Model file for the job. Use its own axes, mm. Give positions to 0.01 mm unless a question says otherwise; leave off trailing zeros. Order: outer loops, then holes, each group sorted by start corner. A loop starts at its lowest first (then second) coordinate and runs counter-clockwise, first axis right, second up. Notation, with made-up numbers: (77.5, 5.25) - (126.5, 5.25) arc R18 ccw to (126.5, 20.25) - close; hole circle Ø11 at (-19, -19). An arc over 180 degrees is marked (long way). Use CSV: the item, a comma, the result in double quotes. Start each with the question number.
(1) Band-saw the part on A-A, the plane x = 0. Give the cut face in (y, z), then the cut area to 3 significant figures.
(2) Band-saw the part on B-B, the plane y = -280. Give the cut face in (x, z).
(3) Probe L1, parallel to Y at x = 0, z = 12.5; L2, parallel to X at y = 269.5, z = 15.5; L3, parallel to Y at x = -280, z = 14.75. List the from-to ranges inside material, lowest first.
(4) Drop flat-ended pins along their axis: pin 1 Ø6 at (y, z) = (71.5, 3.5) entering from -X; pin 2 Ø1 at (y, z) = (-243, 13.5) entering from -X; pin 3 Ø2 at (y, z) = (221, 7) entering from -X. Give the stop position or say it passes through.
(5) Band-saw the part on D-D, the plane z = 23.5. Count the separate pieces of the cut face and the enclosed holes in it, then the cut area to 3 significant figures.
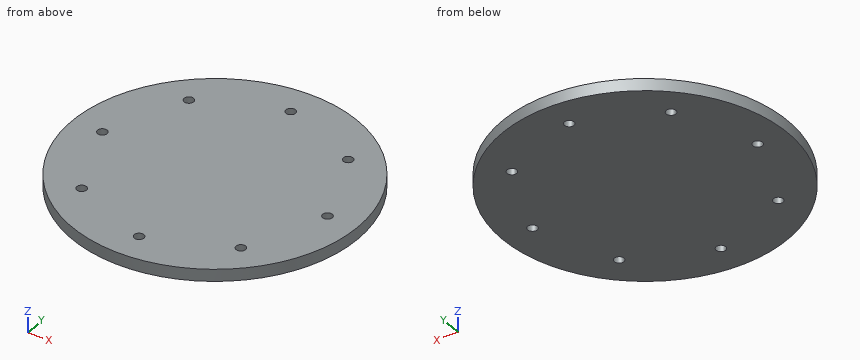
from build123d import *

# Parameters (mm, degrees)
F0_R     = 355
F0_R_2   = 12
F1_DEPTH = 30


with BuildPart() as f1:
    # F0 (on Top) → F1 (new body)
    with BuildSketch(Plane.XY):
        Circle(F0_R)
        with Locations((-197.989899, -197.989899)):
            Circle(F0_R_2, mode=Mode.SUBTRACT)
        with Locations((0, -280)):
            Circle(F0_R_2, mode=Mode.SUBTRACT)
        with Locations((197.989899, -197.989899)):
            Circle(F0_R_2, mode=Mode.SUBTRACT)
        with Locations((-280, 0)):
            Circle(F0_R_2, mode=Mode.SUBTRACT)
        with Locations((-197.989899, 197.989899)):
            Circle(F0_R_2, mode=Mode.SUBTRACT)
        with BuildLine():
            ThreePointArc((292, 0), (280, -12), (268, 0))
            ThreePointArc((268, 0), (280, 12), (292, 0))
        make_face(mode=Mode.SUBTRACT)
        with Locations((0, 280)):
            Circle(F0_R_2, mode=Mode.SUBTRACT)
        with Locations((197.989899, 197.989899)):
            Circle(F0_R_2, mode=Mode.SUBTRACT)
    extrude(amount=F1_DEPTH)


solid = f1.part
Answer block:
1,outline,"(-355, 0) - (-292, 0) - (-292, 30) - (-355, 30) - close; (-268, 0) - (268, 0) - (268, 30) - (-268, 30) - close; (292, 0) - (355, 0) - (355, 30) - (292, 30) - close"
1,area,"19,900 mm2"
2,outline,"(-218.23, 0) - (-12, 0) - (-12, 30) - (-218.23, 30) - close; (12, 0) - (218.23, 0) - (218.23, 30) - (12, 30) - close"
3,L1,"y = -355 to -292, -268 to 268, 292 to 355"
3,L2,"x = -231.07 to -5.81, 5.81 to 231.07"
3,L3,"y = -218.23 to -12, 12 to 218.23"
4,pin 1,"stops at x = -348.33"
4,pin 2,"stops at x = -259.27"
4,pin 3,"stops at x = -278.61"
5,separate pieces,"1"
5,enclosed holes,"8"
5,area,"392,000 mm2"
